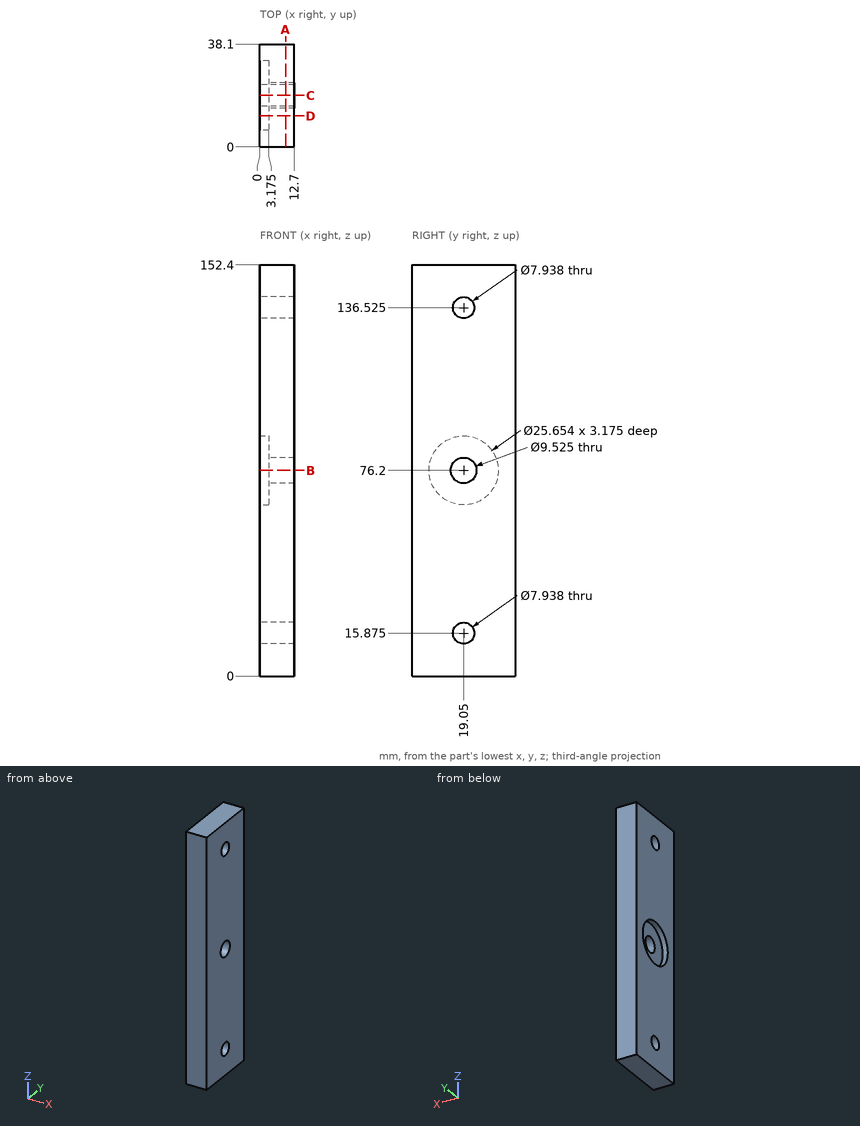
Geometry check sheet. Reference: drawing and pictorial views, mm from the part's lowest x, y, z. Coordinates: 2 decimals unless noted, no trailing zeros. Write each loop counter-clockwise with the first axis right and the second up, starting at its lowest first coordinate (ties: lowest second). Pieces come first, ordered by that corner, then holes. Notation, with made-up numbers: (72.5, 6.5) - (90.5, 6.5) arc R28 ccw to (90.5, 34.5) - close; hole circle Ø10 at (2.25, 79.5). An arc over 180 degrees is marked (long way). Write item = value, one per line.
Q1. Cross-section at D-D (y = 11.5). Enter the section's corners in (x, z) (1 decimal).
Answer:
outline = (0, 0) - (12.7, 0) - (12.7, 152.4) - (0, 152.4) - (0, 86.6) - (3.2, 86.6) - (3.2, 65.8) - (0, 65.8) - close
Q2. Go/stop test with a flat-tipped pin: pin 1 Ø12.5 at (y, z) = (19.05, 76.2) entering from -X (1 decimal). Record where the tip stops, or that it passes through.
Answer:
pin_1 = 3.2
Q3. Material ranges on L1, parallel to Z at x = 10.75, y = 19; L2, parallel to X at y = 14.5, z = 73 (1 decimal); L3, parallel to Y at x = 2.05, z = 76.2, recorded low to high. Write a range as from..to.
Answer:
L1 = 0..11.91, 19.84..71.44, 80.96..132.56, 140.49..152.4
L2 = 3.2..12.7
L3 = 0..6.22, 31.88..38.1
Q4. Cross-section at C-C (y = 19.05). Enter the section's corners in (x, z) (1 decimal), plus the area to 3 significant figures.
Answer:
outline = (0, 0) - (12.7, 0) - (12.7, 11.9) - (0, 11.9) - close; (0, 19.8) - (12.7, 19.8) - (12.7, 71.4) - (3.2, 71.4) - (3.2, 63.4) - (0, 63.4) - close; (0, 89) - (3.2, 89) - (3.2, 81) - (12.7, 81) - (12.7, 132.6) - (0, 132.6) - close; (0, 140.5) - (12.7, 140.5) - (12.7, 152.4) - (0, 152.4) - close
area = 1,560 mm²
Q5. Cross-section at A-A (x = 9.5). Give the number of separate pieces and of enclosed holes in the cut face, plus the area to 3 significant figures.
Answer:
separate_pieces = 1
enclosed_holes = 3
area = 5,640 mm²
Q6. Cross-section at B-B (z = 76.2). Enter the section's corners in (x, y) (1 decimal), plus the area to 3 significant figures.
Answer:
outline = (0, 0) - (12.7, 0) - (12.7, 14.3) - (3.2, 14.3) - (3.2, 6.2) - (0, 6.2) - close; (0, 31.9) - (3.2, 31.9) - (3.2, 23.8) - (12.7, 23.8) - (12.7, 38.1) - (0, 38.1) - close
area = 312 mm²
